Verification items for the finished model (mm, model axes). A direction names the side the tool comes from. Round coordinates to 2 decimals unless told otherwise and drop trailing zeros. Order: outer loops, then holes, each group sorted by start corner. A loop starts at its lowest first (then second) coordinate and runs counter-clockwise, first axis right, second up. Notation, with made-up numbers: (67.25, 68) -> (98.25, 68) arc R36 ccw to (98.25, 107) -> close; hole circle Ø7 at (54, 18). An arc over 180 degrees is marked (long way). Write item = value, one per line. Start each with the question number.
from build123d import *

# Parameters (mm, degrees)
SKETCH1_W           = 290
SKETCH1_H           = 114
BOSS_EXTRUDE1_DEPTH = 10
SKETCH2_W           = 290
SKETCH2_H           = 2
CUT_EXTRUDE1_DEPTH  = 7
SKETCH3_R           = 4
CUT_EXTRUDE2_DEPTH  = 4
SKETCH4_R           = 10
CUT_EXTRUDE3_DEPTH  = 10


with BuildPart() as part:
    # Sketch1 → Boss-Extrude1 (new body)
    with BuildSketch(Plane(origin=(0, 0, 0), x_dir=(1, 0, 0), z_dir=(0, 1, 0))):
        with Locations((145, 57)):
            Rectangle(SKETCH1_W, SKETCH1_H)
    extrude(amount=BOSS_EXTRUDE1_DEPTH)

    # Sketch2 → Cut-Extrude1 (cut)
    with BuildSketch(Plane(origin=(0, 10, 0), x_dir=(1, 0, 0), z_dir=(0, 1, 0))):
        with Locations((145, 113)):
            Rectangle(SKETCH2_W, SKETCH2_H)
        with Locations((145, 1)):
            Rectangle(SKETCH2_W, SKETCH2_H)
    extrude(amount=-CUT_EXTRUDE1_DEPTH, mode=Mode.SUBTRACT)

    # Sketch3 → Cut-Extrude2 (cut)
    with BuildSketch(Plane(origin=(290, 0, 0), x_dir=(0, 0, -1), z_dir=(1, 0, 0))):
        with Locations((22, 5)):
            Circle(SKETCH3_R)
        with Locations((92, 5)):
            Circle(SKETCH3_R)
    extrude(amount=-CUT_EXTRUDE2_DEPTH, mode=Mode.SUBTRACT)

    # Sketch4 → Cut-Extrude3 (cut)
    with BuildSketch(Plane(origin=(0, 10, 0), x_dir=(1, 0, 0), z_dir=(0, 1, 0))):
        with Locations(Location((30, 57, 0), (0, 0, 270))):
            Circle(SKETCH4_R)
    extrude(amount=-CUT_EXTRUDE3_DEPTH, mode=Mode.SUBTRACT)


solid = part.part
(1) Scan lines: line 1 along Z through (x, y) = (144, 5.25); line 2 along X through (y, z) = (4.5, -57); line 3 along X through (y, z) = (2.5, -56). Record each from-to range of solid material in increasing order. Write a range as from..to.
(2) Set-up check for faces 1 (the flat face through (143, 10, -58)), 2 (the cylindrical face through (288, 2.6, -18.8)), 3 (the flat face through (143, 7, -112)): record each of +Z, -Z, +X, -X, +Y, -Y from which the full face is reachable in a straight line by a thin tool's end or side.
(3) Draft check along Y on faces 4 (the flat face through (143, 7, -2)), 5 (the flat face through (286, 5, -22)), 6 (the flat face through (286, 5, -92)), 7 (the flat face through (143, 0, -58)). Enter one of: +Y half, -Y half, draft (parallel to the pull), parting line (faces both ways), or undercut.
(4) Cross-section at D-D (x = 216). Enter the section's corners in (y, z).
(5) Cross-section at C-C (x = 30). Enter the section's corners in (y, z), and give its area (3 significant figures).
(6) Depth check by flat-ended pin: pin 1 (1 mm diameter, centred on x = 102, z = -1, fed in from +Y); pin 2 (2 mm diameter, centred on x = 176.5, y = 7, fed in from +Z); pin 3 (2.5 mm diameter, centred on y = 4, z = -93.5, fed in from +X). Enter the tip coordinate at first touch or a pass-through.
(7) Cross-section at A-A (z = -57). Enter the section's corners in (x, y).
(8) Cross-section at B-B (y = 5). Enter the section's corners in (x, z), and give its area (3 significant figures).
Outcome:
q1.line_1 = -112..-2
q1.line_2 = 0..20, 40..290
q1.line_3 = 0..20.05, 39.95..290
q2.face_1 = +Z, -Z, +X, -X, +Y
q2.face_2 = +X
q2.face_3 = -Z, +X, -X, +Y
q3.face_4 = draft
q3.face_5 = undercut
q3.face_6 = undercut
q3.face_7 = -Y half
q4.outline = (0, -114) -> (3, -114) -> (3, -112) -> (10, -112) -> (10, -2) -> (3, -2) -> (3, 0) -> (0, 0) -> close
q5.outline = (0, -114) -> (3, -114) -> (3, -112) -> (10, -112) -> (10, -67) -> (0, -67) -> close; (0, -47) -> (10, -47) -> (10, -2) -> (3, -2) -> (3, 0) -> (0, 0) -> close
q5.area = 912 mm^2
q6.pin_1 = 3
q6.pin_2 = -2
q6.pin_3 = 286
q7.outline = (0, 0) -> (20, 0) -> (20, 10) -> (0, 10) -> close; (40, 0) -> (290, 0) -> (290, 10) -> (40, 10) -> close
q8.outline = (0, -112) -> (290, -112) -> (290, -96) -> (286, -96) -> (286, -88) -> (290, -88) -> (290, -26) -> (286, -26) -> (286, -18) -> (290, -18) -> (290, -2) -> (0, -2) -> close; hole circle Ø20 at (30, -57)
q8.area = 31,500 mm^2
